Geometry: final body of the model. Coordinates: model frame, mm. A direction names the side the tool comes from. Round coordinates to 2 decimals unless told otherwise and drop trailing zeros. Write each loop counter-clockwise with the first axis right and the second up, starting at its lowest first coordinate (ties: lowest second). Pieces come first, ordered by that corner, then holes. Notation, with made-up numbers: M -25.5,19.5 L 18.5,19.5 A26 cw 18.5,35.5 Z; hole C -5,45.5 d3. An arc over 180 degrees is marked long. Answer as CSV lines item,"result". Start each with the question number.
Q1. First-contact query: pin 1 (0.6 mm diameter, centred on x = 24.5, y = 2.5, fed in from +Z); pin 2 (4 mm diameter, centred on x = 9, z = 9, fed in from +Y); pin 3 (1.4 mm diameter, centred on y = 2.5, z = 4.5, fed in from -X). Flat tips, straight axial feed; report the tip coordinate or a pass-through.
Q2. Reachability of faces 5 (the flat face through (21, 1, 26.67)), 6 (the flat face through (24, 3, 2.381)), 7 (the cylindrical face through (4.763, 1.114, 23.53)) from +Z, -Z, +X, -X, +Y, -Y: full face, straight path, thin tool, end or side. Return the list, or none.
Q3. Section query D-D on x = 31.5. Output: boundary loops of the cut face in (y, z), and give its area (3 significant figures).
Q4. Section query C-C on z = 11. Output: boundary loops of the cut face in (x, y).
Q5. Ray query, probe 1 along Z at (x, y) = (17, 1.95); probe 2 along X at (y, z) = (2.9, 5); probe 3 along Z at (x, y) = (21.5, 1.6). Return the intervals inside material, ascending.
Q6. Mould query, pull axis Z, two halves, no side actions, for faces 1 (the flat face through (20.193, 3, 4)), 2 (the flat face through (0, 1, 13)), 3 (the cylindrical face through (39.49, 1.11, 1.81)), 4 (the flat face through (21, 1, 21.908)). Classes: pulls with the +Z half, pulls with the -Z half, needs draft (parallel to the pull), parting line crosses it, or undercut.
```python
from build123d import *

# Parameters (mm, degrees)
F1_DEPTH  = 2.2606
F2_W      = 25.9304894134
F2_H      = 7.9375
F3_DEPTH  = 0.396875
F4_W      = 14.351
F4_H      = 1.778
F5_DEPTH  = 1.27
F6_SIZE   = 0.79375
F10_DEPTH = 2.2606
F12_DEPTH = 6.35
F13_W     = 0.635
F13_H     = 1.778
F14_DEPTH = 27.8775


# Not quite as in the source:
# - a feature names something its author has since deleted; it is built from what else it names


with BuildPart() as f1:
    # F0 (on Front) → F1 (new body)
    with BuildSketch(Plane.XZ):
        with BuildLine():
            ThreePointArc((0, 6.35), (1.8598719395, 1.8598719395), (6.35, 0))
            Line((6.35, 0), (35.052, 0))
            ThreePointArc((35.052, 0), (39.5421280605, 1.8598719395), (41.402, 6.35))
            Line((41.402, 6.35), (41.402, 20.32))
            ThreePointArc((41.402, 20.32), (39.5421280605, 24.8101280605), (35.052, 26.67))
            Line((35.052, 26.67), (6.35, 26.67))
            ThreePointArc((6.35, 26.67), (1.8598719395, 24.8101280605), (0, 20.32))
            Line((0, 20.32), (0, 6.35))
        make_face()
    extrude(amount=-F1_DEPTH)

    # F2 (on face) → F3 (cut)
    with BuildSketch(Plane(origin=(0, 2.2606, 0), x_dir=(-1, 0, 0), z_dir=(0, 1, 0))):
        with Locations((-20.4992552933, 10.57275)):
            Rectangle(F2_W, F2_H)
    extrude(amount=-F3_DEPTH, mode=Mode.SUBTRACT)

    # F4 (on face) → F5 (join)
    with BuildSketch(Plane(origin=(0, 2.2606, 0), x_dir=(-1, 0, 0), z_dir=(0, 1, 0))):
        with Locations((-20.701, -0.889)):
            Rectangle(F4_W, F4_H)
        Polygon((-21.209, 2.38125), (-26.8605, 2.38125), (-26.8605, 6.2865), (-27.8765, 6.2865), (-27.8765, 0), (-13.5255, 0), (-13.5255, 6.2865), (-14.5415, 6.2865), (-14.5415, 2.38125), (-20.193, 2.38125), (-20.193, 6.2865), (-21.209, 6.2865), align=None)
    extrude(amount=F5_DEPTH)

    # F6
    f6_edges = [f1.edges().sort_by_distance(p)[0] for p in [
        (27.3685, 3.5306, 6.2865),
        (20.701, 3.5306, 6.2865),
        (14.0335, 3.5306, 6.2865),
    ]]
    chamfer(f6_edges, length=F6_SIZE)

    # F9 (on Front) → F10 (cut, through all)
    with BuildSketch(Plane.XZ):
        with BuildLine():
            Line((6.35, 21.9075), (35.052, 21.9075))
            ThreePointArc((35.052, 21.9075), (36.6395, 23.495), (35.052, 25.0825))
            Line((35.052, 25.0825), (6.35, 25.0825))
            ThreePointArc((6.35, 25.0825), (4.7625, 23.495), (6.35, 21.9075))
        make_face()
    extrude(amount=-F10_DEPTH, mode=Mode.SUBTRACT)

    # F11 (on face) → F12 (join, symmetric)
    with BuildSketch(Plane.YZ.offset(20.701)):
        with BuildLine():
            Line((2.2606, 26.67), (2.2606, 25.1591298729))
            Line((2.2606, 25.1591298729), (2.8956, 25.1591298729))
            ThreePointArc((2.8956, 25.1591298729), (3.3446128061, 25.3451170669), (3.5306, 25.7941298729))
            Line((3.5306, 25.7941298729), (3.5306, 26.67))
            Line((3.5306, 26.67), (3.5306, 28.575))
            Line((3.5306, 28.575), (2.8956, 28.575))
            Line((2.8956, 28.575), (2.8956, 26.67))
            Line((2.8956, 26.67), (2.2606, 26.67))
        make_face()
    extrude(amount=F12_DEPTH, both=True)

    # F13 (on face) → F14 (cut, through all)
    with BuildSketch(Plane(origin=(13.5255, 0, 0), x_dir=(0, -1, 0), z_dir=(-1, 0, 0))):
        with Locations((-2.5781, -0.889)):
            Rectangle(F13_W, F13_H)
    extrude(amount=-F14_DEPTH, mode=Mode.SUBTRACT)


solid = f1.part
```
Entries:
1,pin 1,"stops at z = 26.67"
1,pin 2,"stops at y = 2.26"
1,pin 3,"stops at x = 0.11"
2,face 5,"+Z, +X, -X, -Y"
2,face 6,"+Y"
2,face 7,"+Y, -Y"
3,outline,"M 0,0 L 2.26,0 L 2.26,6.6 L 1.86,6.6 L 1.86,14.54 L 2.26,14.54 L 2.26,21.91 L 0,21.91 Z; M 0,25.08 L 2.26,25.08 L 2.26,26.67 L 0,26.67 Z"
3,area,"50.0 mm^2"
4,outline,"M 0,0 L 41.4,0 L 41.4,2.26 L 33.46,2.26 L 33.46,1.86 L 7.53,1.86 L 7.53,2.26 L 0,2.26 Z"
5,probe 1,"z = 0 to 6.6, 14.54 to 21.91, 25.08 to 26.67"
5,probe 2,"x = 13.53 to 14.54, 20.19 to 21.21, 26.86 to 27.88"
5,probe 3,"z = 0 to 21.91, 25.08 to 26.67"
6,face 1,"undercut"
6,face 2,"needs draft"
6,face 3,"pulls with the -Z half"
6,face 4,"undercut"
